```python
from build123d import *

# Parameters (mm, degrees)
SKETCH1_W               = 8
SKETCH1_H               = 8
BOSS_EXTRUDE1_DEPTH     = 3
CUT_EXTRUDE1_DEPTH      = 12.704699911
CUT_EXTRUDE1_DEPTH_BACK = 12.704699911
CUT_EXTRUDE2_DEPTH      = 11
SKETCH4_R               = 1.8
CUT_EXTRUDE3_DEPTH      = 0.8
SKETCH5_W               = 8
SKETCH5_H               = 1
BOSS_EXTRUDE2_DEPTH     = 2
FILLET1_R               = 4
CUT_EXTRUDE4_DEPTH      = 0.4


with BuildPart() as part:
    # Sketch1 → Boss-Extrude1 (new body)
    with BuildSketch(Plane(origin=(0, 0, 0), x_dir=(1, 0, 0), z_dir=(0, 1, 0))):
        with Locations((4, 4)):
            Rectangle(SKETCH1_W, SKETCH1_H)
    extrude(amount=BOSS_EXTRUDE1_DEPTH)

    # Sketch2 → Cut-Extrude1 (cut, two sides: drawn at the far end of the back side and taken through both)
    with BuildSketch(Plane.XY.offset(-CUT_EXTRUDE1_DEPTH_BACK)):
        Polygon((0, 0), (0.6, 3), (0, 3), align=None)
        Polygon((8, 0), (7.4, 3), (8, 3), align=None)
    extrude(amount=CUT_EXTRUDE1_DEPTH + CUT_EXTRUDE1_DEPTH_BACK, mode=Mode.SUBTRACT)

    # Sketch3 → Cut-Extrude2 (cut)
    with BuildSketch(Plane(origin=(0, 0, 0), x_dir=(0, 0, -1), z_dir=(1, 0, 0))):
        Polygon((0, 0), (0.6, 3), (0, 3), align=None)
        Polygon((8, 3), (7.4, 3), (8, 0), align=None)
    extrude(amount=CUT_EXTRUDE2_DEPTH, mode=Mode.SUBTRACT)

    # Sketch4 → Cut-Extrude3 (cut)
    with BuildSketch(Plane.XZ):
        with Locations(Location((4, -3.75, 0), (0, 0, 270))):
            Circle(SKETCH4_R)
    extrude(amount=-CUT_EXTRUDE3_DEPTH, mode=Mode.SUBTRACT)

    # Sketch5 → Boss-Extrude2 (add)
    with BuildSketch(Plane.XZ):
        with Locations((4, -7.5)):
            Rectangle(SKETCH5_W, SKETCH5_H)
    extrude(amount=BOSS_EXTRUDE2_DEPTH)

    # Fillet1
    # the kernel refuses this fillet: 4 mm, written as the material it takes off along each edge
    with BuildSketch(Plane(origin=(8, -2, -16.660254038), x_dir=(0, 1, 0), z_dir=(0, 0, 1)), Plane(origin=(0, -2, 1.660254038), x_dir=(0, 1, 0), z_dir=(0, 0, -1))) as fillet1_piece_1:
        with BuildLine():
            CenterArc((4, 3.464101615), FILLET1_R, 180, 60)
            Line((0, 3.464101615), (-0.08, 3.464101615))
            Line((-0.08, 3.464101615), (-0.08, 0))
            Line((-0.08, 0), (0, -0.08))
            ThreePointArc((0, -0.08), (1, -0.08), (1.96, -0.069282032))
            Line((1.96, -0.069282032), (2, 0))
        make_face()
    extrude(amount=18.320508076, mode=Mode.SUBTRACT)

    # Sketch6 → Cut-Extrude4 (cut)
    with BuildSketch(Plane(origin=(0, 3, 0), x_dir=(1, 0, 0), z_dir=(0, 1, 0))):
        with BuildLine():
            add(Edge.make_bspline(
                [(5.284087955, 2.773445367), (5.333545491, 2.739545524), (5.432652736, 2.671614118), (5.590291823, 2.583736248), (5.752942084, 2.503846486), (5.865979951, 2.460876102), (5.92270975, 2.439310751)],
                knots=[0, 0, 0, 0, 0.994855506, 1.99357661, 2.993045438, 4, 4, 4, 4], degree=3))
            Line((5.92270975, 2.439310751), (5.628639237, 1.875208187))
            add(Edge.make_bspline(
                [(5.628639237, 1.875208187), (5.568520037, 1.893818156), (5.447325875, 1.93133395), (5.332925255, 1.986187111), (5.275273852, 2.013829982)],
                knots=[0, 0, 0, 0, 0.992113803, 2, 2, 2, 2], degree=3))
            add(Edge.make_bspline(
                [(5.275273852, 2.013829982), (5.26961656, 2.016684314), (5.253233801, 2.024950075), (5.223476786, 2.045298413), (5.178074812, 2.072724498), (5.118973761, 2.11071311), (5.045578888, 2.157800121), (4.95765273, 2.213934729), (4.856407872, 2.280704114), (4.783596416, 2.327731001), (4.744825134, 2.35277229)],
                knots=[0, 0, 0, 0, 0.241377655, 0.698997227, 1.371388316, 2.263975901, 3.376788369, 4.695767198, 6.240533187, 8, 8, 8, 8], degree=3))
            add(Edge.make_bspline(
                [(4.744825134, 2.35277229), (4.712670389, 2.339001865), (4.648050063, 2.311327899), (4.547788838, 2.27725121), (4.444978029, 2.248544986), (4.339982896, 2.224200245), (4.232359046, 2.206111381), (4.122258624, 2.192239309), (4.00937299, 2.18410397), (3.933139287, 2.183304154), (3.894664878, 2.182900495)],
                knots=[0, 0, 0, 0, 0.961025642, 1.931341354, 2.907359807, 3.893838693, 4.891829695, 5.905170566, 6.942759923, 8, 8, 8, 8], degree=3))
            add(Edge.make_bspline(
                [(3.894664878, 2.182900495), (3.821683976, 2.184676763), (3.679027131, 2.188148859), (3.471015208, 2.212756542), (3.275562804, 2.255408477), (3.091812023, 2.313667662), (2.920867424, 2.390147666), (2.761229426, 2.482594503), (2.615108223, 2.593406711), (2.480490537, 2.71918809), (2.361392609, 2.861354588), (2.257130725, 3.017424584), (2.168806746, 3.186880722), (2.097587685, 3.370615377), (2.041301668, 3.567142879), (2.002926315, 3.777850586), (1.978227581, 4.001488849), (1.975427333, 4.155321196), (1.973991801, 4.234182546)],
                knots=[0, 0, 0, 0, 1.098101164, 2.146474535, 3.146072545, 4.104420533, 5.041773038, 5.958565538, 6.874115049, 7.795336865, 8.725215067, 9.658214839, 10.614563411, 11.594512188, 12.618591104, 13.685899083, 14.813688224, 16, 16, 16, 16], degree=3))
            add(Edge.make_bspline(
                [(1.973991801, 4.234182546), (1.97543059, 4.313040679), (1.978227497, 4.466335509), (2.002757559, 4.689542909), (2.042412611, 4.899497801), (2.098124704, 5.096337583), (2.170410456, 5.279545107), (2.259079723, 5.449017762), (2.363505524, 5.605417057), (2.484015277, 5.747270094), (2.617919267, 5.874338646), (2.764464989, 5.984327234), (2.9219486, 6.078236158), (3.090996271, 6.154643933), (3.272074664, 6.212871015), (3.463805003, 6.255387163), (3.667248709, 6.280295733), (3.806454886, 6.283712517), (3.877837955, 6.285464598)],
                knots=[0, 0, 0, 0, 1.193283781, 2.319662245, 3.393996131, 4.424093603, 5.411284417, 6.369670503, 7.313761776, 8.251713527, 9.181123148, 10.102053383, 11.01932051, 11.951118596, 12.903560284, 13.893239571, 14.919681386, 16, 16, 16, 16], degree=3))
            add(Edge.make_bspline(
                [(3.877837955, 6.285464598), (3.948708316, 6.284176334), (4.086935049, 6.281663683), (4.288489067, 6.254790298), (4.478939684, 6.214016744), (4.658513444, 6.155241629), (4.826290277, 6.078911265), (4.983143341, 5.98623667), (5.128157857, 5.876434989), (5.26137487, 5.750578969), (5.380523981, 5.609215368), (5.486073462, 5.454669187), (5.572731816, 5.285035211), (5.645736122, 5.103191508), (5.700157026, 4.90736457), (5.740330715, 4.69867705), (5.764520815, 4.476471411), (5.76739165, 4.323719862), (5.768863596, 4.245400495)],
                knots=[0, 0, 0, 0, 1.078752742, 2.104017338, 3.091035458, 4.041673215, 4.975566109, 5.892967701, 6.810684895, 7.740128604, 8.678185021, 9.621404646, 10.583875016, 11.573429805, 12.6009998, 13.674031063, 14.80742018, 16, 16, 16, 16], degree=3))
            add(Edge.make_bspline(
                [(5.768863596, 4.245400495), (5.767275795, 4.16278925), (5.764189157, 4.002195454), (5.737326284, 3.768977018), (5.693780668, 3.550562854), (5.648918616, 3.41330904), (5.627036673, 3.346362034)],
                knots=[0, 0, 0, 0, 1.083667057, 2.106616435, 3.076482036, 4, 4, 4, 4], degree=3))
            add(Edge.make_bspline(
                [(5.627036673, 3.346362034), (5.607421404, 3.297050064), (5.567517691, 3.196733787), (5.488642668, 3.051933408), (5.394797316, 2.909076479), (5.321514211, 2.819296637), (5.284087955, 2.773445367)],
                knots=[0, 0, 0, 0, 0.948216854, 1.928975575, 2.942311585, 4, 4, 4, 4], degree=3))
        make_face()
        with BuildLine():
            add(Edge.make_bspline(
                [(4.642261032, 3.185304341), (4.671182259, 3.216922768), (4.72909393, 3.280235293), (4.800707281, 3.388678336), (4.863230922, 3.50497094), (4.912388312, 3.632014464), (4.951923574, 3.76787431), (4.97951585, 3.913560578), (4.996652709, 4.068707035), (4.998621406, 4.175375245), (4.999632827, 4.230176136)],
                knots=[0, 0, 0, 0, 0.906820982, 1.815812261, 2.745108282, 3.70056618, 4.696560745, 5.740060838, 6.83895416, 8, 8, 8, 8], degree=3))
            add(Edge.make_bspline(
                [(4.999632827, 4.230176136), (4.998745764, 4.286560817), (4.997027382, 4.395786947), (4.982794262, 4.554398979), (4.957747484, 4.70183414), (4.925058455, 4.838707416), (4.88052022, 4.963910999), (4.826807351, 5.078388614), (4.763835344, 5.182421929), (4.690056733, 5.274294514), (4.608907177, 5.355063587), (4.522159409, 5.426414517), (4.428546166, 5.486139657), (4.328544236, 5.534184829), (4.222990468, 5.571989212), (4.111634776, 5.59943433), (3.994225982, 5.615495039), (3.913944994, 5.6176829), (3.873030263, 5.618797931)],
                knots=[0, 0, 0, 0, 1.335693338, 2.587451293, 3.768164612, 4.876224393, 5.916940853, 6.910477009, 7.867661778, 8.790666633, 9.694493319, 10.576027549, 11.446684429, 12.318352473, 13.199023277, 14.098364444, 15.030842682, 16, 16, 16, 16], degree=3))
            add(Edge.make_bspline(
                [(3.873030263, 5.618797931), (3.831841607, 5.617719084), (3.751279942, 5.615608947), (3.633755604, 5.599158788), (3.522145798, 5.573035665), (3.416723766, 5.534932642), (3.316536446, 5.486796326), (3.222573421, 5.427181815), (3.134847786, 5.356951252), (3.053289548, 5.276692152), (2.980446173, 5.184790487), (2.915694165, 5.082568667), (2.862164439, 4.968850144), (2.819178201, 4.84427298), (2.784825228, 4.709477379), (2.760087026, 4.563739976), (2.745835322, 4.407279692), (2.744110931, 4.299383286), (2.74322257, 4.243797931)],
                knots=[0, 0, 0, 0, 0.980107447, 1.917010591, 2.819119613, 3.703969481, 4.579773866, 5.459928929, 6.346604172, 7.250235365, 8.177620171, 9.131899985, 10.124404622, 11.161948974, 12.264485933, 13.431998172, 14.677033863, 16, 16, 16, 16], degree=3))
            add(Edge.make_bspline(
                [(2.74322257, 4.243797931), (2.744089067, 4.187408458), (2.745771696, 4.077907007), (2.760333697, 3.91913972), (2.783941374, 3.771215716), (2.817547327, 3.634196218), (2.86051391, 3.507924697), (2.913437174, 3.392577112), (2.976036542, 3.288297709), (3.048513511, 3.196032652), (3.128245057, 3.114861766), (3.213441608, 3.04409835), (3.303411645, 2.983479498), (3.39857486, 2.934226809), (3.498956775, 2.896402137), (3.604207339, 2.869103357), (3.714939061, 2.852831885), (3.790443662, 2.850669982), (3.82895975, 2.849567162)],
                knots=[0, 0, 0, 0, 1.356840463, 2.634818045, 3.833173645, 4.958776583, 6.025986406, 7.038359119, 8.007356852, 8.946032033, 9.855123386, 10.740685277, 11.607120956, 12.460971081, 13.313368256, 14.183325659, 15.073285775, 16, 16, 16, 16], degree=3))
            add(Edge.make_bspline(
                [(3.82895975, 2.849567162), (3.857844622, 2.850073951), (3.914741814, 2.851072222), (3.998801079, 2.862293633), (4.080683558, 2.878515583), (4.133570622, 2.895033243), (4.159889237, 2.903253059)],
                knots=[0, 0, 0, 0, 1.028828871, 2.026578908, 3.017950568, 4, 4, 4, 4], degree=3))
            add(Edge.make_bspline(
                [(4.159889237, 2.903253059), (4.119539232, 2.924336443), (4.039635796, 2.966086993), (3.916101198, 3.019284802), (3.792319766, 3.067214804), (3.708133251, 3.09310976), (3.666299493, 3.105977418)],
                knots=[0, 0, 0, 0, 1.021704821, 2.023239566, 3.017713044, 4, 4, 4, 4], degree=3))
            Line((3.666299493, 3.105977418), (3.889857186, 3.56751588))
            add(Edge.make_bspline(
                [(3.889857186, 3.56751588), (3.955233958, 3.544923565), (4.086618506, 3.49952088), (4.276409331, 3.409366748), (4.463555304, 3.306758821), (4.582244486, 3.226093623), (4.642261032, 3.185304341)],
                knots=[0, 0, 0, 0, 0.979271047, 1.967993817, 2.972492781, 4, 4, 4, 4], degree=3))
        make_face(mode=Mode.SUBTRACT)
    extrude(amount=-CUT_EXTRUDE4_DEPTH, mode=Mode.SUBTRACT)


solid = part.part
```
Work out the finished part from the listing and answer in its coordinate system (mm). A direction names the side the tool comes from. Coordinates: 2 decimals unless noted, no trailing zeros. Order: outer loops, then holes, each group sorted by start corner. A loop starts at its lowest first (then second) coordinate and runs counter-clockwise, first axis right, second up. Notation, with made-up numbers: M 73,3 L 131,3 A19 ccw 131,21 Z; hole C 42.25,24.5 d2. An arc over 180 degrees is marked long. Use CSV: the item, a comma, the result in double quotes.
1) Section B-B on x = 7 is taken. Write down the section's boundary in (y, z).
Worked out:
outline,"M -1.15,-8 L 0,-8 L 3,-7.4 L 3,-0.6 L 0,0 L 0,-7 L -1.15,-7 Z"
2) For faces 1 (the face through (3, 0, -2)), 2 (the face through (4, 0.8, -4)), 3 (the face through (4, -1, -8)), determine the directions among +Z, -Z, +X, -X, +Y, -Y from which every point of the face is accessible in a straight line to the end or side of a thin tool.
Worked out:
face 1,"+Z, +X, -X, -Y"
face 2,"-Y"
face 3,"-Z, +X, -X, +Y, -Y"
3) Section D-D on y = 2.5 is taken. Write down the section's boundary in (x, z), plus the area to 3 significant figures.
Worked out:
outline,"M 0.5,-7.5 L 7.5,-7.5 L 7.5,-0.5 L 0.5,-0.5 Z"
area,"49.0 mm^2"
4) Consider line 1 (Y direction, x = 3, z = -6.75); line 2 (X direction, y = 0.65, z = -3.75); line 3 (Z direction, x = 3.5, y = -0.15). Determine where each line is inside the solid, lowest interval first. Write a range as [from, to].
Worked out:
line 1,"y = [0, 3]"
line 2,"x = [0.13, 2.2], [5.8, 7.87]"
line 3,"z = [-8, -7]"
5) Section A-A on y = 0.4 is taken. Write down the section's boundary in (x, z).
Worked out:
outline,"M 0.08,-7.92 L 7.92,-7.92 L 7.92,-0.08 L 0.08,-0.08 Z; hole C 4,-3.75 d3.6"
6) Determine the mould class of faces 4 (the face through (4, -1, -7)), 5 (the face through (7.7, 1.5, -4.1)), 6 (the face through (1.49, -1.48, -7.49)), 7 (the face through (4.4, 2.6, -3.1)) for opening direction X: released by +X, released by -X, zero draft, split by the parting line, or undercut.
Worked out:
face 4,"zero draft"
face 5,"released by +X"
face 6,"released by -X"
face 7,"undercut"
7) A flat-ended cylindrical pin translates along its axis: pin 1 Ø3 at (x, z) = (3.5, -3) entering from -Y. Find the tip coordinate at first contact, or state that the pin passes through.
Worked out:
pin 1,"stops at y = 0"
8) Section C-C on z = -6.75 is taken. Write down the section's boundary in (x, y).
Worked out:
outline,"M 0,0 L 8,0 L 7.4,3 L 0.6,3 Z"
